Build history of the part. All positions in model axes, mm. Face numbers are marked on the shaded views. Give positions to 0.01 mm unless a question says otherwise; leave off trailing zeros. Order: outer loops, then holes, each group sorted by start corner. A loop starts at its lowest first (then second) coordinate and runs counter-clockwise, first axis right, second up. Notation, with made-up numbers: (65, 70.25) -> (97, 70.25) arc R12 cw to (97, 76.25) -> close; hole circle Ø9 at (44.5, 25). An arc over 180 degrees is marked (long way). One line per item, written item: value. Start each with the question number.
(1) Probe line 1 (Z direction, x = 27, y = 16.75); line 2 (X direction, y = 23.5, z = -11); line 3 (X direction, y = 19.5, z = -4). List the from-to ranges inside material, lowest first.
(2) Saw through at B-B on y = 5.5. Give the cut face in (x, z), plus the area to 3 significant figures.
(3) Saw through at D-D on z = -8.5. Count the separate pieces of the cut face and the enclosed holes in it, plus the area to 3 significant figures.
(4) Saw through at C-C on x = 4.5. Give the cut face in (y, z).
(5) Pin check, flat tips, straight feed: pin 1 (3 mm diameter, centred on x = -4, y = 9.5, fed in from +Z); pin 2 (13 mm diameter, centred on y = 15.5, z = 4, fed in from -X); pin 3 (4 mm diameter, centred on x = -14.5, z = 2.5, fed in from -Y); pin 4 (3.5 mm diameter, centred on y = 10.5, z = 22, fed in from +X). Stop position of each tip, or through.
(6) Saw through at A-A on x = -33.5. Give the cut face in (y, z).
(7) Two-plate mould, pull along X, no slides. Class the marked faces 1, 2 and 3: +X half, -X half, draft (parallel to the pull), parting line (faces both ways), or undercut.
```python
from build123d import *

# Parameters (mm, degrees)
ESQUISSE1_W          = 72
ESQUISSE1_H          = 33
BOSS_EXTRU_1_DEPTH   = 26
ESQUISSE3_R          = 1.6
BOSS_EXTRU_2_DEPTH   = 25.689186
BOSS_EXTRU_2_2_DEPTH = 25.689186
ESQUISSE4_R          = 1.6
R_VOLUTION1_ANGLE    = 180


with BuildPart() as part:
    # Esquisse1 → Boss.-Extru.1 (new body)
    with BuildSketch(Plane(origin=(0, 0, 0), x_dir=(1, 0, 0), z_dir=(0, 1, 0))):
        Rectangle(ESQUISSE1_W, ESQUISSE1_H)
    extrude(amount=BOSS_EXTRU_1_DEPTH)



with BuildPart() as body_2:
    # Esquisse3 → Boss.-Extru.2 (new body)
    with BuildSketch(Plane.ZY.offset(10.310814339)):
        with Locations((21.300154865, 18.67433682)):
            Circle(ESQUISSE3_R)
    extrude(amount=BOSS_EXTRU_2_DEPTH)


with BuildPart() as body_3:
    # Esquisse3 → Boss.-Extru.2 2 (new body)
    with BuildSketch(Plane.ZY.offset(10.310814339)):
        with Locations((21.300154865, 10.80733682)):
            Circle(ESQUISSE3_R)
    extrude(amount=BOSS_EXTRU_2_2_DEPTH)


with BuildPart() as part_1:
    add(part.part)

    add(body_2.part)  # R_volution1 merges body 2

    add(body_3.part)  # R_volution1 merges body 3
    # Esquisse4 → R_volution1 (revolve)
    with BuildSketch(Plane.ZY.offset(36)):
        with Locations((21.300154865, 18.67433682)):
            Circle(ESQUISSE4_R)
        with Locations((21.300154865, 10.80733682)):
            Circle(ESQUISSE4_R)
    revolve(axis=Axis((-36, 26, 3.300154865), (0, -1, 0)), revolution_arc=R_VOLUTION1_ANGLE)


solid = part_1.part
```
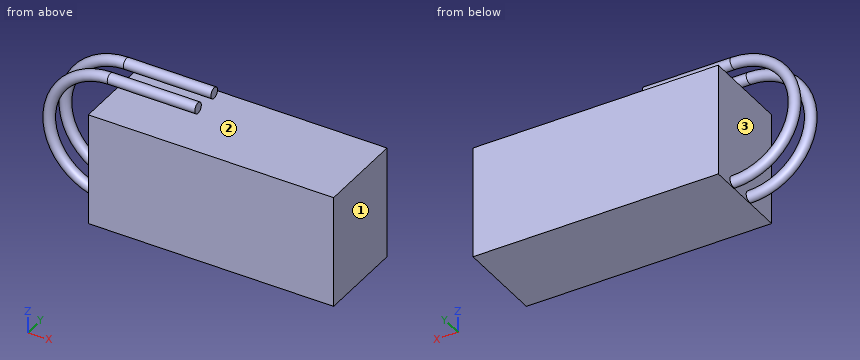
Results below:
1. line 1: z = -16.5 to 16.5
1. line 2: x = -36 to 36
1. line 3: x = -53.94 to -50.94, -36 to 36
2. outline: (-36, -16.5) -> (36, -16.5) -> (36, 16.5) -> (-36, 16.5) -> close
2. area: 2,380 mm²
3. separate pieces: 3
3. enclosed holes: 0
3. area: 1,890 mm²
4. outline: (0, -16.5) -> (26, -16.5) -> (26, 16.5) -> (0, 16.5) -> close
5. pin 1: stops at z = 16.5
5. pin 2: stops at x = -55.6
5. pin 3: stops at y = 0
5. pin 4: stops at x = -10.31
6. outline: (0, -16.5) -> (26, -16.5) -> (26, 16.5) -> (0, 16.5) -> close; circle Ø3.2 at (10.81, 21.3); circle Ø3.2 at (18.67, 21.3)
7. face 1: +X half
7. face 2: draft
7. face 3: undercut
